Read the model definition and answer for the solid it produces. Units are mm, in the model's axes. A direction names the side the tool comes from. Coordinates: 2 decimals unless noted, no trailing zeros. Loops run counter-clockwise (first coordinate to the right, second up) from the corner with the lowest first, then second, coordinate; pieces in that order, holes last. Notation, with made-up numbers: (34.5, 5) -> (70.5, 5) arc R24 cw to (70.5, 15) -> close; hole circle Ø2 at (67, 23.25). An arc over 180 degrees is marked (long way). Answer as a JSON object with one key per item and string values. Group by question number.
1) Section A-A, the plane y = 105 is taken. Give the vertices of the cut face in (x, z), plus the area to 3 significant figures.
2) Section D-D, the plane y = 224 is taken. Give the vertices of the cut face in (x, z), plus the area to 3 significant figures.
3) Consider probe 1 along Y at (x, z) = (0, 51); probe 2 along Z at (x, y) = (17.5, 41); probe 3 along Y at (x, z) = (-1.5, 38). Determine where each line is inside the solid, lowest interval first. Write a range as [from, to].
4) Section B-B, the plane x = 0 is taken. Give the vertices of the cut face in (y, z) (3 decimals).
5) Flat-ended cylindrical pins translate along their axes: P1, Ø1, axis at x = 6.5, z = 11.5, coming from the +Y side; P2, Ø2, axis at x = -4, z = 17, coming from the +Y side; P3, Ø23, axis at x = 0, y = 105, coming from the -Z side; P4, Ø5, axis at y = 200.5, z = 25, coming from the -X side. Find the tip coordinate at first contact, or state that the pin passes through.
6) Determine the mould class of faces 4 (the face through (0, 105, 50.5)), 5 (the face through (-30, 107, 43)), 6 (the face through (-14, 107, 55.5)) for opening direction X: released by +X, released by -X, zero draft, split by the parting line, or undercut.
7) Section C-C, the plane z = 19 is taken. Give the vertices of the cut face in (x, y) (3 decimals).
8) Which of the six approach directions +Z, -Z, +X, -X, +Y, -Y give full straight-line access (tool end or side, diameter ignored) to faces 1 (the face through (-1.302, 114.915, 53.035)), 2 (the face through (1.89, 205.57, 15.97)), 3 (the face through (0, -10, 0))?
Autodesk Inventor part; units mm, degrees
ref_plane "YZ Plane" through (0, 0, 0) normal (1, 0, 0) x (0, 1, 0)
ref_plane "XZ Plane" through (0, 0, 0) normal (0, 1, 0) x (-1, 0, 0)
ref_plane "XY Plane" through (0, 0, 0) normal (0, 0, 1) x (1, 0, 0)
sketch "Эскиз1" plane through (0, 0, 0) normal (0, 0, 1) x (1, 0, 0)
  circle A0 centre (0, -10) radius 9
  circle A1 centre (0, -10) radius 14.5552
  point P0 (0, 0)
extrude "Выдавливание1" add sketch "Эскиз1" along normal blind 31.5 contours A0 | A1
sketch "Эскиз2" plane through (0, -10, 31.5) normal (0, 0, 1) x (1, 0, 0)
  line L0 (0, 0) -> (0, 230) construction
  line L1 (30, 0) -> (30, 230)
  line L2 (-30, 230) -> (-30, 0)
  arc A0 (-30, 0) -> (30, 0) centre (0, 0) ccw
  arc A1 (30, 230) -> (-30, 230) centre (0, 230) ccw
  circle A2 centre (0, 0) radius 14.5552
  point P0 (0, 10)
  point P1 (0, 115)
  dimension "d4" = 230
  dimension "d5" = 30
extrude "Выдавливание2" add sketch "Эскиз2" along normal blind 24 contours A0 L2 A1 L1 | A2
sketch "Эскиз3" plane through (0, -10, 31.5) normal (0, 0, -1) x (-1, 0, 0)
  circle A0 centre (0, 230) radius 14.555
  arc A1 (30, 230) -> (-30, 230) centre (0, 230) ccw
  point P0 (0, 10)
  dimension "d6" = 29.11
extrude "Выдавливание3" add sketch "Эскиз3" along normal up to surface (31.5 mm away)
sketch "Эскиз4" plane through (0, -10, 55.5) normal (0, 0, 1) x (1, 0, 0)
  arc A0 (30, 230) -> (-30, 230) centre (0, 230) ccw
  line L0 (-30, 230) -> (-30, 0)
  arc A1 (-30, 0) -> (30, 0) centre (0, 0) ccw
  line L1 (30, 0) -> (30, 230)
  circle A2 centre (0, 115) radius 10
  point P0 (0, 10)
  dimension "d9" = 20
extrude "Выдавливание4" cut sketch "Эскиз4" against normal blind 5 contours A2
properties part number "Колено"
Determined:
{
 "1": {"outline": "(-30, 31.5) -> (30, 31.5) -> (30, 55.5) -> (10, 55.5) -> (10, 50.5) -> (-10, 50.5) -> (-10, 55.5) -> (-30, 55.5) -> close", "area": "1,340 mm²"},
 "2": {"outline": "(-29.73, 31.5) -> (-13.99, 31.5) -> (-13.99, 0) -> (13.99, 0) -> (13.99, 31.5) -> (29.73, 31.5) -> (29.73, 55.5) -> (-29.73, 55.5) -> close", "area": "2,310 mm²"},
 "3": {"probe 1": "[-40, 95], [115, 250]", "probe 2": "[31.5, 55.5]", "probe 3": "[-39.96, 249.96]"},
 "4": {"outline": "(-40, 31.5) -> (-24.555, 31.5) -> (-24.555, 0) -> (4.555, 0) -> (4.555, 31.5) -> (205.445, 31.5) -> (205.445, 0) -> (234.555, 0) -> (234.555, 31.5) -> (250, 31.5) -> (250, 55.5) -> (115, 55.5) -> (115, 50.5) -> (95, 50.5) -> (95, 55.5) -> (-40, 55.5) -> close"},
 "5": {"P1": "y = 233.26", "P2": "y = 234.24", "P3": "z = 31.5", "P4": "through"},
 "6": {"face 4": "undercut", "face 5": "released by -X", "face 6": "zero draft"},
 "7": {"outline": "circle Ø29.11 at (0, -10); circle Ø29.11 at (0, 220)"},
 "8": {"face 1": "+Z", "face 2": "-Z", "face 3": "-Z, +X, -X, +Y, -Y"}
}
